CAD build for the part. Positions are in the model's coordinates, mm. Face numbers are marked on the shaded views. A direction names the side the tool comes from. Round coordinates to 2 decimals unless told otherwise and drop trailing zeros. Loops run counter-clockwise (first coordinate to the right, second up) from the corner with the lowest first, then second, coordinate; pieces in that order, holes last.
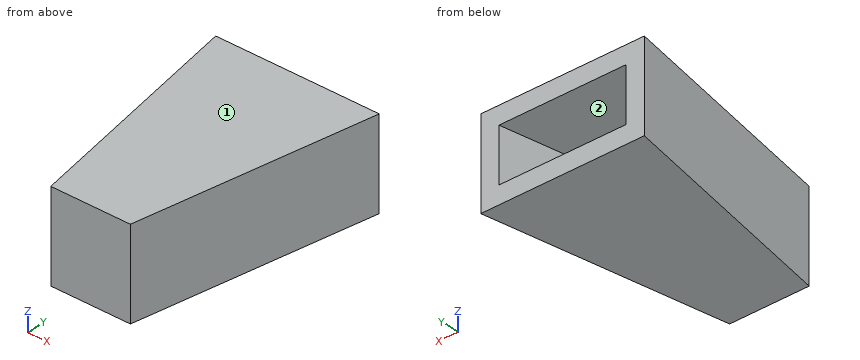
```python
from build123d import *

# Parameters (mm, degrees)
EXTRUDE_1_DEPTH = 7.5
SHELL_1_T       = -1.5


with BuildPart() as part:
    # 草图1 → 凸台-拉伸1 (new body)
    with BuildSketch(Plane.XY):
        Polygon((-22.163477656, 55), (-15.358999723, 55), (-8.487673684, 55), (-11.922964888, 35.089989422), (-18.582368801, 35.089989422), align=None)
    extrude(amount=EXTRUDE_1_DEPTH)

    # 抽壳1
    shell_1_openings = [part.faces().sort_by_distance(p)[0] for p in [
        (-15.32557567, 55, 3.75),
    ]]
    offset(amount=SHELL_1_T, openings=shell_1_openings, kind=Kind.INTERSECTION)


solid = part.part
```
Item 1: Probe line 1 (Z direction, x = -17.75, y = 47.25); line 2 (Y direction, x = -14.25, z = 2.5); line 3 (X direction, y = 41.75, z = 3.75). List the from-to ranges inside material, lowest first.
Answers follow:
line 1: z = 0 to 1.5, 6 to 7.5
line 2: y = 35.09 to 36.59
line 3: x = -19.78 to -18.26, -12.3 to -10.77
Item 2: Cut at D-D, the plane y = 42.5. Give the cut face in (x, z), plus the area to 3 significant figures.
Answers follow:
outline: (-19.92, 0) - (-10.64, 0) - (-10.64, 7.5) - (-19.92, 7.5) - close; hole (-18.39, 1.5) - (-12.17, 1.5) - (-12.17, 6) - (-18.39, 6) - close
area: 41.5 mm2
Item 3: Flat gauge pin, fed straight in: P1, Ø4.5, axis at x = -15, z = 3.5, coming from the +Y side. Where does the tip first touch, or does it go through?
Answers follow:
P1: stops at y = 55
Item 4: Cut at C-C, the plane z = 3. Give the cut face in (x, y), plus the area to 3 significant figures.
Answers follow:
outline: (-22.16, 55) - (-18.58, 35.09) - (-11.92, 35.09) - (-8.49, 55) - (-10.01, 55) - (-13.19, 36.59) - (-17.33, 36.59) - (-20.64, 55) - close
area: 66.5 mm2
Item 5: Cut at A-A, the plane x = -14.75. Give the cut face in (y, z), plus the area to 3 significant figures.
Answers follow:
outline: (35.09, 0) - (55, 0) - (55, 1.5) - (36.59, 1.5) - (36.59, 6) - (55, 6) - (55, 7.5) - (35.09, 7.5) - close
area: 66.5 mm2
Item 6: 3-axis set-ups, long thin cutter, end or side, ignore diameter. For the marked faces 1 and 2: which of +Z, -Z, +X, -X, +Y, -Y reach the whole face in a straight line?
Answers follow:
face 1: +Z, +X, -X, +Y, -Y
face 2: +Y
Item 7: Cut at B-B, the plane y = 48. Give the cut face in (x, z), plus the area to 3 significant figures.
Answers follow:
outline: (-20.9, 0) - (-9.7, 0) - (-9.7, 7.5) - (-20.9, 7.5) - close; hole (-19.38, 1.5) - (-11.22, 1.5) - (-11.22, 6) - (-19.38, 6) - close
area: 47.3 mm2
